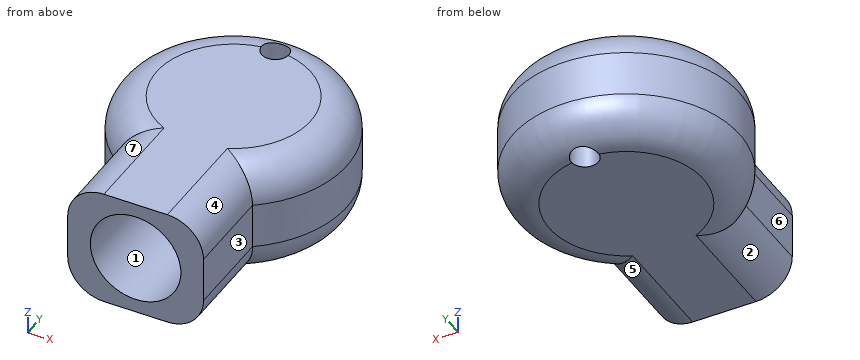
from build123d import *

# Parameters (mm, degrees)
F1_DEPTH = 16.51
F2_R     = 5.08
F4_D     = 3.81
F6_D     = 12.7
F6_DEPTH = 28.575
F6_TIP   = 3.8154649308


with BuildPart() as f1:
    # F0 (on Top) → F1 (new body)
    with BuildSketch(Plane.XY):
        with BuildLine():
            Line((9.525, -25.4), (9.525, -12.7))
            ThreePointArc((9.525, -12.7), (0, 15.875), (-9.525, -12.7))
            Line((-9.525, -12.7), (-9.525, -25.4))
            Line((-9.525, -25.4), (9.525, -25.4))
        make_face()
    extrude(amount=F1_DEPTH)

    # F2
    f2_edges = [f1.edges().sort_by_distance(p)[0] for p in [
        (0, 15.875, 16.51),
        (-9.525, -19.05, 16.51),
        (9.525, -19.05, 16.51),
        (0, 15.875, 0),
        (-9.525, -19.05, 0),
        (9.525, -19.05, 0),
    ]]
    fillet(f2_edges, radius=F2_R)

    # F4 (through all)
    with Locations(Plane.XY.offset(16.51)):
        with Locations((0, 10.795)):
            Hole(F4_D / 2)

    # F6
    with Locations(Plane.XZ.offset(25.4)):
        with Locations((0, 8.255)):
            Hole(F6_D / 2, depth=F6_DEPTH)
            with Locations((0, 0, -(F6_DEPTH + F6_TIP / 2))):  # 118° drill point
                Cone(0, F6_D / 2, F6_TIP, mode=Mode.SUBTRACT)


solid = f1.part
Model file for the job. Use its own axes, mm. Face numbers are marked on the shaded views. A direction names the side the tool comes from. Round coordinates to 2 decimals unless told otherwise and drop trailing zeros. Order: outer loops, then holes, each group sorted by start corner. A loop starts at its lowest first (then second) coordinate and runs counter-clockwise, first axis right, second up.
(1) Pull direction X, two halves, no side cores. Call the marked faces 1, 2 and 3: released by +X, released by -X, zero draft, split by the parting line, or undercut.
(2) Band-saw the part on C-C (y = -20.5). List the corners of the cut face in (x, z) (3 decimals), then the cut area to 3 significant figures.
(3) Band-saw the part on A-A (y = 0). List the corners of the cut face in (x, z) (3 decimals).
(4) 3-axis set-ups, long thin cutter, end or side, ignore diameter. For the marked faces 4, 5, 6 and 7: which of +Z, -Z, +X, -X, +Y, -Y reach the whole face in a straight line?
(5) Drill centre lines: line 1 (X direction, y = -21.5, z = 11.5); line 2 (Z direction, x = -7.5, y = 8); line 3 (Y direction, x = 1, z = 13.25). Where is each one in solid material? Low to high.
(6) Pin check, flat tips, straight feed: pin 1 (2 mm diameter, centred on x = -10.5, z = 7, fed in from +Y); pin 2 (3 mm diameter, centred on x = -12, z = 11, fed in from +Y); pin 3 (6 mm diameter, centred on y = 11, z = 4, fed in from +X). Stop position of each tip, or through.
(7) Band-saw the part on B-B (z = 15.75). List the corners of the cut face in (x, y) (3 decimals), then the cut area to 3 significant figures.
Verdict:
1. face 1: undercut
1. face 2: released by -X
1. face 3: released by +X
2. outline: (-9.525, 5.08) arc R5.08 ccw to (-4.445, 0) - (4.445, 0) arc R5.08 ccw to (9.525, 5.08) - (9.525, 11.43) arc R5.08 ccw to (4.445, 16.51) - (-4.445, 16.51) arc R5.08 ccw to (-9.525, 11.43) - close; hole circle Ø12.7 at (0, 8.255)
2. area: 166 mm2
3. outline: (-15.875, 5.08) arc R5.08 ccw to (-10.795, 0) - (10.795, 0) arc R5.08 ccw to (15.875, 5.08) - (15.875, 11.43) arc R5.08 ccw to (10.795, 16.51) - (-10.795, 16.51) arc R5.08 ccw to (-15.875, 11.43) - close; hole circle Ø12.7 at (0, 8.255)
4. face 4: +Z, +X, -Y
4. face 5: -Z, +X, -Y
4. face 6: +Z, -Z, -X, -Y
4. face 7: +Z, -X, -Y
5. line 1: x = -9.52 to -5.46, 5.46 to 9.52
5. line 2: z = 0 to 16.51
5. line 3: y = 3.93 to 9.17, 12.42 to 15.51
6. pin 1: stops at y = 12.72
6. pin 2: stops at y = 11.91
6. pin 3: stops at x = 13.65
7. outline: (-7.118, -25.4) - (7.118, -25.4) - (7.118, -11.433) arc R13.468 ccw (long way) to (-7.118, -11.433) - close; hole circle Ø3.81 at (0, 10.795)
7. area: 738 mm2
